Input: part model. Units: mm. Frame: model coordinates. Face numbers are marked on the shaded views. A direction names the side the tool comes from. Round coordinates to 2 decimals unless told otherwise and drop trailing zeros. Loops run counter-clockwise (first coordinate to the right, second up) from the corner with the lowest first, then second, coordinate; pieces in that order, holes last. Notation, with made-up numbers: (7, 89) -> (53, 89) arc R26 cw to (53, 107) -> close; hole circle Ø9 at (-35, 80). An arc over 180 degrees is marked (long way). One line per question, with ' | ' between items. Start each with the question number.
Q1. Cut plane D-D on z = -73.5. Return loops of the section in (x, y).
Q2. Cut plane B-B on x = 0. Return loops of the section in (y, z) (3 decimals), and give its area (4 significant figures).
Q3. Mould query, pull axis X, two halves, no side actions, for the marked faces 1, 2 and 3. Classes: pulls with the +X half, pulls with the -X half, needs draft (parallel to the pull), parting line crosses it, or undercut.
Q4. Contact query for a flat-ended pin moving along its axis: P1, Ø4, axis at x = 0, z = -10, coming from the +Y side. Output: stop coordinate, or through.
Q5. Cut plane A-A on y = 0.25. Return loops of the section in (x, z).
Q6. Material intervals for L1, parallel to Y at x = -4.25, z = -57.5; L2, parallel to X at y = 8.9, z = -80 (3 decimals), sorted ascending.
Q7. Access query for the marked faces 4 and 5. Directions: +Z, -Z, +X, -X, +Y, -Y. A direction counts if a zero-diameter tool reaches every point of the face in a straight line with its end or side. Return the directions, or none.
Q8. Cut plane C-C on z = -10. Return loops of the section in (x, y) (3 decimals).
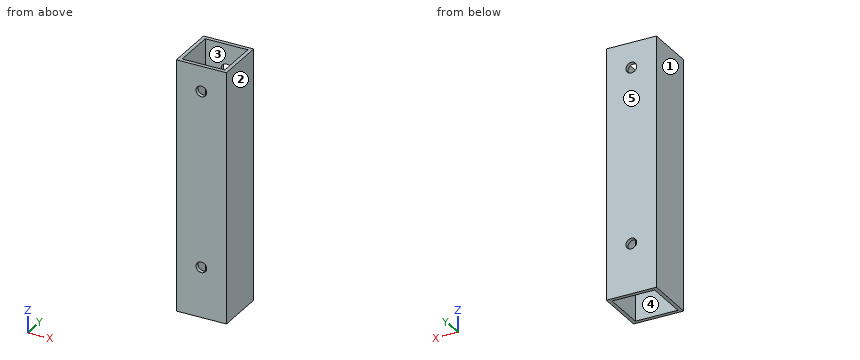
from build123d import *

# Parameters (mm, degrees)
SKETCH1_W           = 20
SKETCH1_H           = 20
SKETCH1_W_2         = 17
SKETCH1_H_2         = 17
BOSS_EXTRUDE1_DEPTH = 100
SKETCH2_R           = 2.125
CUT_EXTRUDE1_DEPTH  = 103.46950766


with BuildPart() as part:
    # Sketch1 → Boss-Extrude1 (new body)
    with BuildSketch(Plane.XY):
        Rectangle(SKETCH1_W, SKETCH1_H)
        Rectangle(SKETCH1_W_2, SKETCH1_H_2, mode=Mode.SUBTRACT)
    extrude(amount=-BOSS_EXTRUDE1_DEPTH)

    # Sketch2 → Cut-Extrude1 (cut, through all)
    with BuildSketch(Plane(origin=(0, 10, 0), x_dir=(1, 0, 0), z_dir=(0, 1, 0))):
        with Locations(Location((0, 10, 0), (0, 0, 270))):
            Circle(SKETCH2_R)
        with Locations(Location((0, 80, 0), (0, 0, 270))):
            Circle(SKETCH2_R)
        with Locations((0, 150)):
            Circle(SKETCH2_R)
    extrude(amount=-CUT_EXTRUDE1_DEPTH, mode=Mode.SUBTRACT)


solid = part.part
Results:
1) outline: (-10, -10) -> (10, -10) -> (10, 10) -> (-10, 10) -> close; hole (-8.5, -8.5) -> (8.5, -8.5) -> (8.5, 8.5) -> (-8.5, 8.5) -> close
2) outline: (-10, -100) -> (-8.5, -100) -> (-8.5, -82.125) -> (-10, -82.125) -> close; (-10, -77.875) -> (-8.5, -77.875) -> (-8.5, -12.125) -> (-10, -12.125) -> close; (-10, -7.875) -> (-8.5, -7.875) -> (-8.5, 0) -> (-10, 0) -> close; (8.5, -100) -> (10, -100) -> (10, -82.125) -> (8.5, -82.125) -> close; (8.5, -77.875) -> (10, -77.875) -> (10, -12.125) -> (8.5, -12.125) -> close; (8.5, -7.875) -> (10, -7.875) -> (10, 0) -> (8.5, 0) -> close | area: 274.5 mm^2
3) face 1: pulls with the -X half | face 2: pulls with the +X half | face 3: undercut
4) P1: through
5) outline: (-10, -100) -> (-8.5, -100) -> (-8.5, 0) -> (-10, 0) -> close; (8.5, -100) -> (10, -100) -> (10, 0) -> (8.5, 0) -> close
6) L1: -10 to -8.5, 8.5 to 10 | L2: -10 to -2.125, 2.125 to 10
7) face 4: +Z, -Z | face 5: +Z, -Z, +X, -X, +Y
8) outline: (-10, -10) -> (-2.125, -10) -> (-2.125, -8.5) -> (-8.5, -8.5) -> (-8.5, 8.5) -> (-2.125, 8.5) -> (-2.125, 10) -> (-10, 10) -> close; (2.125, -10) -> (10, -10) -> (10, 10) -> (2.125, 10) -> (2.125, 8.5) -> (8.5, 8.5) -> (8.5, -8.5) -> (2.125, -8.5) -> close
